from build123d import *

# Parameters (mm, degrees)
SKETCH1_R           = 1
BOSS_EXTRUDE1_DEPTH = 6


with BuildPart() as part:
    # Sketch1 → Boss-Extrude1 (new body)
    with BuildSketch(Plane(origin=(0, 0, 0), x_dir=(1, 0, 0), z_dir=(0, 1, 0))):
        with BuildLine():
            Line((0, 0), (100, 0))
            Line((100, 0), (100, 70))
            ThreePointArc((100, 70), (50, 120), (0, 70))
            Line((0, 70), (0, 0))
        make_face()
        with Locations(Location((22, 95, 0), (0, 0, 270))):
            Circle(SKETCH1_R, mode=Mode.SUBTRACT)
        with Locations(Location((78, 95, 0), (0, 0, 270))):
            Circle(SKETCH1_R, mode=Mode.SUBTRACT)
        with Locations(Location((30, 25, 0), (0, 0, 270))):
            Circle(SKETCH1_R, mode=Mode.SUBTRACT)
        with Locations(Location((70, 25, 0), (0, 0, 270))):
            Circle(SKETCH1_R, mode=Mode.SUBTRACT)
    extrude(amount=BOSS_EXTRUDE1_DEPTH)


solid = part.part
Can you work these out from the model? Positions are in its coordinate system, mm. Coordinates: 2 decimals unless noted, no trailing zeros. Loops run counter-clockwise (first coordinate to the right, second up) from the corner with the lowest first, then second, coordinate; pieces in that order, holes last. Notation, with made-up numbers: (17.5, -23) - (46.5, -23) arc R17 cw to (46.5, -5) - close; hole circle Ø1 at (17.25, -2). An arc over 180 degrees is marked (long way). Put each result on its own line as item: value. Start each with the question number.
Item 1: Suppose I cut it at A-A (y = 2.75). Please give me the cut outline in (x, z).
Item 2: For pin 1 (2.5 mm diameter, centred on x = 30, z = -25, fed in from -Y); pin 2 (1.8 mm diameter, centred on x = 22, z = -95, fed in from -Y), each with a flat end and sliding along its axis, tell me the tip position at first contact or that it passes through.
Item 3: Suppose I cut it at B-B (x = 12). Please give me the cut outline in (y, z), and give its area (3 significant figures).
Item 4: If I drill on line 1 along X through (y, z) = (3.15, -25); line 2 along X through (y, z) = (4.4, -95); line 3 along Z through (x, y) = (55, 0.8), over which ranges is the centre line in solid material (lowest first)?
Item 5: Suppose I cut it at C-C (x = 64.5). Please give me the cut outline in (y, z), and give its area (3 significant figures).
Here are the results:
1. outline: (0, -70) arc R50 ccw to (100, -70) - (100, 0) - (0, 0) - close; hole circle Ø2 at (22, -95); hole circle Ø2 at (30, -25); hole circle Ø2 at (70, -25); hole circle Ø2 at (78, -95)
2. pin 1: y = 0
2. pin 2: through
3. outline: (0, -102.5) - (6, -102.5) - (6, 0) - (0, 0) - close
3. area: 615 mm²
4. line 1: 0 to 29, 31 to 69, 71 to 100
4. line 2: 6.7 to 21, 23 to 77, 79 to 93.3
4. line 3: -119.75 to 0
5. outline: (0, -117.85) - (6, -117.85) - (6, 0) - (0, 0) - close
5. area: 707 mm²
